Work out the finished part from the listing and answer in its coordinate system (mm). A direction names the side the tool comes from. Round coordinates to 2 decimals unless told otherwise and drop trailing zeros. Order: outer loops, then holes, each group sorted by start corner. A loop starts at its lowest first (then second) coordinate and runs counter-clockwise, first axis right, second up. Notation, with made-up numbers: (85, -17) - (112, -17) arc R27 cw to (112, 4) - close; hole circle Ø6 at (79, 19.25). An arc over 180 degrees is marked (long way). Put each result on its own line as item: value.
```python
from build123d import *

# Parameters (mm, degrees)
BOSS_EXTRUDE1_DEPTH = 5.08
SKETCH2_W           = 36.285714285
SKETCH2_H           = 5.08
SKETCH2_W_2         = 36.285714286
CUT_EXTRUDE1_DEPTH  = 5.08
SKETCH3_W           = 36.285714285
SKETCH3_H           = 5.08
SKETCH3_W_2         = 36.285714286
CUT_EXTRUDE2_DEPTH  = 5.08
SKETCH4_W           = 36.285714285
SKETCH4_H           = 5.08
SKETCH4_W_2         = 36.285714286
CUT_EXTRUDE3_DEPTH  = 5.08
SKETCH5_R           = 21.59
CUT_EXTRUDE4_DEPTH  = 5.08
SKETCH6_W           = 17.78
SKETCH6_H           = 5.08
SKETCH6_W_2         = 5.08
SKETCH6_H_2         = 20.32
CUT_EXTRUDE5_DEPTH  = 11.16


with BuildPart() as part:
    # Sketch1 → Boss-Extrude1 (new body)
    with BuildSketch(Plane(origin=(0, 0, 0), x_dir=(1, 0, 0), z_dir=(0, 1, 0))):
        Polygon((0, 0), (-254, 0), (-127, 219.970452561), align=None)
    extrude(amount=BOSS_EXTRUDE1_DEPTH)

    # Sketch2 → Cut-Extrude1 (cut)
    with BuildSketch(Plane(origin=(0, 0, 0), x_dir=(-0.5, 0, -0.866025404), z_dir=(0.866025404, 0, -0.5))):
        with Locations((199.571428572, 2.54)):
            Rectangle(SKETCH2_W, SKETCH2_H)
        with Locations((127, 2.54)):
            Rectangle(SKETCH2_W_2, SKETCH2_H)
        with Locations((54.428571428, 2.54)):
            Rectangle(SKETCH2_W, SKETCH2_H)
    extrude(amount=-CUT_EXTRUDE1_DEPTH, mode=Mode.SUBTRACT)

    # Sketch3 → Cut-Extrude2 (cut)
    with BuildSketch(Plane(origin=(-190.5, 0, -109.985226281), x_dir=(-0.5, 0, 0.866025404), z_dir=(-0.866025404, 0, -0.5))):
        with Locations((-72.571428572, 2.54)):
            Rectangle(SKETCH3_W, SKETCH3_H)
        with Locations((0, 2.54)):
            Rectangle(SKETCH3_W_2, SKETCH3_H)
        with Locations((72.571428572, 2.54)):
            Rectangle(SKETCH3_W, SKETCH3_H)
    extrude(amount=-CUT_EXTRUDE2_DEPTH, mode=Mode.SUBTRACT)

    # Sketch4 → Cut-Extrude3 (cut)
    with BuildSketch(Plane.XY):
        with Locations((-199.571428572, 2.54)):
            Rectangle(SKETCH4_W, SKETCH4_H)
        with Locations((-127, 2.54)):
            Rectangle(SKETCH4_W_2, SKETCH4_H)
        with Locations((-54.428571428, 2.54)):
            Rectangle(SKETCH4_W, SKETCH4_H)
    extrude(amount=-CUT_EXTRUDE3_DEPTH, mode=Mode.SUBTRACT)

    # Sketch5 → Cut-Extrude4 (cut)
    with BuildSketch(Plane(origin=(0, 5.08, 0), x_dir=(1, 0, 0), z_dir=(0, 1, 0))):
        with Locations((-127, 73.66)):
            Circle(SKETCH5_R)
    extrude(amount=-CUT_EXTRUDE4_DEPTH, mode=Mode.SUBTRACT)

    # Sketch6 → Cut-Extrude5 (cut, through all)
    with BuildSketch(Plane(origin=(0, 10.16, 0), x_dir=(1, 0, 0), z_dir=(0, 1, 0))):
        with Locations((-149.055874493, 149.882969593)):
            Rectangle(SKETCH6_W, SKETCH6_H)
        with Locations((-104.605874493, 149.36329839)):
            Rectangle(SKETCH6_W, SKETCH6_H)
        with Locations((-99.525874493, 129.889965056)):
            Rectangle(SKETCH6_W_2, SKETCH6_H_2)
        with Locations((-103.592773819, 109.0579774)):
            Rectangle(SKETCH6_W, SKETCH6_H)
        with Locations((-149.987461319, 109.600384218)):
            Rectangle(SKETCH6_W, SKETCH6_H)
        with Locations((-155.572009554, 129.965942855)):
            Rectangle(SKETCH6_W_2, SKETCH6_H_2)
    extrude(amount=-CUT_EXTRUDE5_DEPTH, mode=Mode.SUBTRACT)


solid = part.part
```
1) Straight lines are drawn through the part: L1, parallel to Z at x = -127, y = 3.05; L2, parallel to X at y = 2.85, z = -132; L3, parallel to Z at x = -101.5, y = 4.2. For each, find the intervals that lie inside material, in ascending order. Write a range as from..to.
Findings below:
L1: z = -219.97..-95.25, -52.07..-5.08
L2: x = -177.79..-158.11, -153.03..-102.07, -96.99..-76.21
L3: z = -165.64..-151.9, -146.82..-140.05, -119.73..-111.6, -106.52..0
2) For faces 5 (the flat face through (-149, 3, -147.343)), 6 (the flat face through (-145.143, 3, -3)), 7 (the flat face through (-81.77, 2.5, -141.63)), determine the directions among +Z, -Z, +X, -X, +Y, -Y from which every point of the face is accessible in a straight line to the end or side of a thin tool.
Findings below:
face 5: +Y, -Y
face 6: +Z, +Y, -Y
face 7: -Z, +X, +Y, -Y
3) A cutting plane is placed at A-A on z = -129. Write down the section's boundary in (x, y).
Findings below:
outline: (-179.52, 0) - (-158.11, 0) - (-158.11, 5.08) - (-179.52, 5.08) - close; (-153.03, 0) - (-102.07, 0) - (-102.07, 5.08) - (-153.03, 5.08) - close; (-96.99, 0) - (-74.48, 0) - (-74.48, 5.08) - (-96.99, 5.08) - close
4) A cutting plane is placed at D-D on x = -66.5. Write down the section's boundary in (y, z).
Findings below:
outline: (0, -105.02) - (5.08, -105.02) - (5.08, -5.08) - (0, -5.08) - close
5) A cutting plane is placed at C-C on y = 2.3. Give the number of separate pieces and of enclosed holes in the cut face, then the cut area to 3 significant figures.
Findings below:
separate pieces: 1
enclosed holes: 7
area: 24,200 mm2
6) A cutting plane is placed at B-B on z = -73.66. Write down the section's boundary in (x, y), then the cut area to 3 significant figures.
Findings below:
outline: (-211.47, 0) - (-148.59, 0) - (-148.59, 5.08) - (-211.47, 5.08) - close; (-105.41, 0) - (-42.53, 0) - (-42.53, 5.08) - (-105.41, 5.08) - close
area: 639 mm2
7) Given pin 1 Ø2.5 at (y, z) = (3.5, -149) entering from -X; pin 2 Ø2.5 at (y, z) = (2.5, -126) entering from +X; pin 3 Ø2.5 at (y, z) = (3.5, -151) entering from +X, each flat-ended and moving along its own axis, determine where each tip first touches the part or whether it passes through.
Findings below:
pin 1: stops at x = -168.7
pin 2: stops at x = -72.57
pin 3: stops at x = -86.46
8) For a pull along X with two mould halves and no side action, classify faces 1 (the flat face through (-9.198, 2.504, -15.932)), 2 (the flat face through (-102.066, 3, -130)), 3 (the flat face through (-153.032, 3, -130)), 4 (the flat face through (-208.77, 2.5, -78.34)) as pulls with the +X half, pulls with the -X half, needs draft (parallel to the pull), parting line crosses it, or undercut.
Findings below:
face 1: pulls with the +X half
face 2: undercut
face 3: undercut
face 4: pulls with the -X half
